```python
from build123d import *

# Parameters (mm, degrees)
F1_DEPTH = 15
F3_DEPTH = 8
F5_START = -1.3
F4_W     = 12.4
F4_H     = 10.6533105238
F5_DEPTH = 12.4
F6_R     = 5
F7_DEPTH = 5
F8_R     = 4.2
F9_DEPTH = 3.5


with BuildPart() as f1:
    # F0 (on Top) → F1 (new body)
    with BuildSketch(Plane.XY):
        with BuildLine():
            Line((7.5, 12.9903810568), (7.5, 29.0473750966))
            ThreePointArc((7.5, 29.0473750966), (0, 30), (-7.5, 29.0473750966))
            Line((-7.5, 29.0473750966), (-7.5, 12.9903810568))
            Line((-7.5, 12.9903810568), (0, 8.6602540378))
            Line((0, 8.6602540378), (7.5, 12.9903810568))
        make_face()
        with BuildLine():
            Line((7.5, 12.9903810568), (21.4057647469, 21.0188780767))
            ThreePointArc((21.4057647469, 21.0188780767), (15, 25.9807621135), (7.5, 29.0473750966))
            Line((7.5, 29.0473750966), (7.5, 12.9903810568))
        make_face()
        with BuildLine():
            Line((15, 0), (28.9057647469, 8.0284970199))
            ThreePointArc((28.9057647469, 8.0284970199), (25.9807621135, 15), (21.4057647469, 21.0188780767))
            Line((21.4057647469, 21.0188780767), (7.5, 12.9903810568))
            Line((7.5, 12.9903810568), (7.5, 4.3301270189))
            Line((7.5, 4.3301270189), (15, 0))
        make_face()
        Polygon((7.5, -4.3301270189), (15, 0), (7.5, 4.3301270189), align=None)
        Polygon((7.5, 4.3301270189), (7.5, 12.9903810568), (0, 8.6602540378), align=None)
        Polygon((5.4903810568, -5.4903810568), (7.5, -4.3301270189), (7.5, 4.3301270189), (0, 8.6602540378), (-7.5, 4.3301270189), (-7.5, 2.0096189432), align=None)
        Polygon((-7.5, 4.3301270189), (0, 8.6602540378), (-7.5, 12.9903810568), align=None)
    extrude(amount=F1_DEPTH)

    # F2 (on face) → F3 (cut)
    with BuildSketch(Plane.XY.offset(15)):
        Polygon((-5.7741669751, 2.3988494278), (-0.4048094716, -0.7011505722), (5.7951905284, 10.0375644347), (0.4258330249, 13.1375644347), align=None)
        Polygon((5.7951905284, 10.0375644347), (-0.4048094716, -0.7011505722), (4.9645480318, -3.8011505722), (11.1645480318, 6.9375644347), align=None)
    extrude(amount=-F3_DEPTH, mode=Mode.SUBTRACT)

    # F4 (on face) → F5 (cut)
    with BuildSketch(Plane.XY.offset(15).offset(F5_START)):
        with Locations((-0.1, 26.3740303584)):
            Rectangle(F4_W, F4_H)
        Polygon((15.1775615166, 15.8064425114), (21.3775615166, 5.0677275044), (35.9265312226, 13.4675790806), (29.7265312226, 24.2062940875), align=None)
    extrude(amount=-F5_DEPTH, mode=Mode.SUBTRACT)

    # F6 (on face) → F7 (join)
    with BuildSketch(Plane(origin=(-1.0048094716, -1.7403810568, 0), x_dir=(0.8660254038, -0.5, 0), z_dir=(-0.5, -0.8660254038, 0))):
        with Locations((0, 7.5)):
            Circle(F6_R)
    extrude(amount=F7_DEPTH)

    # F8 (on face) → F9 (cut)
    with BuildSketch(Plane(origin=(18.2275615166, 10.5236875483, 0), x_dir=(-0.5, 0.8660254038, 0), z_dir=(0.8660254038, 0.5, 0))):
        with Locations((-0.1, 7.5)):
            Circle(F8_R)
    extrude(amount=-F9_DEPTH, mode=Mode.SUBTRACT)


solid = f1.part
```
Input: part model. Units: mm. Frame: model coordinates. A direction names the side the tool comes from. Coordinates: 2 decimals unless noted, no trailing zeros. Write each loop counter-clockwise with the first axis right and the second up, starting at its lowest first coordinate (ties: lowest second). Pieces come first, ordered by that corner, then holes.
1) Section B-B on y = 22. Output: boundary loops of the cut face in (x, z).
2) Set-up query: faces 4 (the flat face through (0, 21.047, 8)), 5 (the flat face through (3, 5, 7)), 6 (the flat face through (-2.539, -0.855, 2.395)), 7 (the flat face through (-7.5, 16, 7)). Return all of +Z, -Z, +X, -X, +Y, -Y with unobstructed straight access to the full face (end or side cutting, diameter ignored); none if empty.
3) Section A-A on z = 2. Output: boundary loops of the cut face in (x, y).
4) Material intervals for line 1 along X through (y, z) = (6.5, 4.5); line 2 along Z through (x, y) = (22.5, 19.5); line 3 along Y through (x, z) = (7, 13), sorted ascending.
5) Pin query (flat end, axial travel): pin 1 Ø10 at (x, y) = (-2.5, 24) entering from -Z; pin 2 Ø5 at (y, z) = (13.5, 3) entering from -X; pin 3 Ø2 at (y, z) = (14, 6) entering from +X; pin 4 Ø4 at (x, z) = (11, 10.5) entering from +Y. Return the tip coordinate at first contact, or that it passes through.
6) Section C-C on x = 24. Output: boundary loops of the cut face in (y, z), and give its area (3 significant figures).
7) Mould query, pull axis X, two halves, no side actions, for faces 1 (the flat face through (18.8, 17.9, 7.6)), 2 (the flat face through (6, 13, 0)), 3 (the flat face through (8.02, 1.49, 11.06)). Classes: pulls with the +X half, pulls with the -X half, needs draft (parallel to the pull), parting line crosses it, or undercut.
8) Section D-D on z = 8.75. Output: boundary loops of the cut face in (x, y).
Check result:
1. outline: (-7.5, 0) - (20.4, 0) - (20.4, 15) - (-7.5, 15) - close; hole (-6.3, 1.3) - (6.1, 1.3) - (6.1, 13.7) - (-6.3, 13.7) - close
2. face 4: +Y
2. face 5: +Z
2. face 6: none
2. face 7: +Z, -Z, -X, +Y
3. outline: (-7.5, 2.01) - (5.49, -5.49) - (28.91, 8.03) arc R30 ccw to (28.55, 9.21) - (21.38, 5.07) - (15.18, 15.81) - (22.39, 19.97) arc R30 ccw to (6.1, 29.37) - (6.1, 21.05) - (-6.3, 21.05) - (-6.3, 29.33) arc R30 ccw to (-7.5, 29.05) - close
4. line 1: x = -7.5 to 16.51, 17.34 to 20.55, 23.86 to 26.26
4. line 2: z = 0 to 1.3, 13.7 to 15
4. line 3: y = -4.62 to -0.28, 9.34 to 29.17
5. pin 1: stops at z = 0
5. pin 2: stops at x = -7.5
5. pin 3: stops at x = 16.53
5. pin 4: stops at y = 28.62
6. outline: (5.2, 0) - (18, 0) - (18, 1.3) - (6.58, 1.3) - (6.58, 13.7) - (18, 13.7) - (18, 15) - (5.2, 15) - close
6. area: 50.5 mm2
7. face 1: pulls with the +X half
7. face 2: needs draft
7. face 3: undercut
8. outline: (-7.7, -3.65) - (0.69, -8.49) - (3.19, -4.16) - (5.49, -5.49) - (28.91, 8.03) arc R30 ccw to (28.55, 9.21) - (21.38, 5.07) - (20.28, 6.96) - (17.25, 5.21) - (13.24, 12.16) - (16.27, 13.91) - (15.18, 15.81) - (22.39, 19.97) arc R30 ccw to (6.1, 29.37) - (6.1, 21.05) - (-6.3, 21.05) - (-6.3, 29.33) arc R30 ccw to (-7.5, 29.05) - (-7.5, 2.01) - (-5.2, 0.68) - close; hole (-5.77, 2.4) - (4.96, -3.8) - (11.16, 6.94) - (0.43, 13.14) - close
